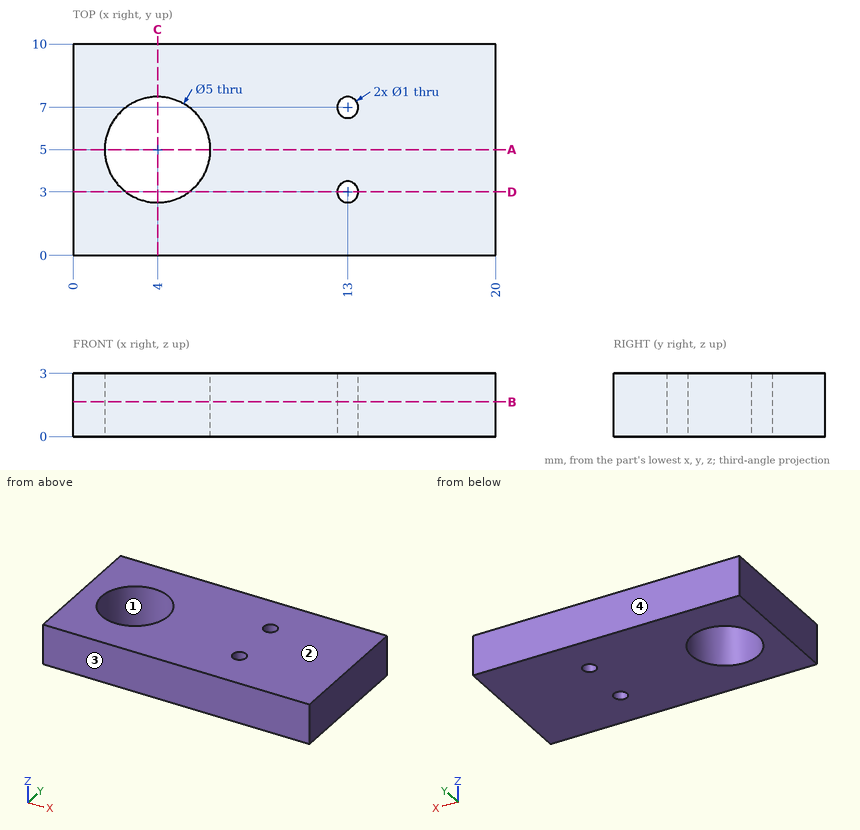
Can you work these out from the drawing? Everything is in mm from the part's minimum corner. Round coordinates to 2 decimals unless told otherwise and drop trailing zeros. Write each loop counter-clockwise with the first axis right and the second up, starting at its lowest first coordinate (ties: lowest second). Pieces come first, ordered by that corner, then holes. Notation, with made-up numbers: (62, 52.25) - (81, 52.25) arc R14 cw to (81, 59.25) - close; hole circle Ø8 at (46.5, -2.75). An arc over 180 degrees is marked (long way). Use a Markdown table: item, result.
Q1. I want a section at C-C (x = 4). List the corners of the cut face in (y, z) for me.
Output values:
| item | result |
|---|---|
| outline | (0, 0) - (2.5, 0) - (2.5, 3) - (0, 3) - close; (7.5, 0) - (10, 0) - (10, 3) - (7.5, 3) - close |
Q2. Please list where these lines run through material, in increasing order: L1, parallel to Y at x = 13, z = 2.2; L2, parallel to Y at x = 4, z = 1.4; L3, parallel to Y at x = 3.25, z = 0.65.
Output values:
| item | result |
|---|---|
| L1 | 0 to 2.5, 3.5 to 6.5, 7.5 to 10 |
| L2 | 0 to 2.5, 7.5 to 10 |
| L3 | 0 to 2.62, 7.38 to 10 |
Q3. I want a section at D-D (y = 3). List the corners of the cut face in (x, z) for me, plus the area to 3 significant figures.
Output values:
| item | result |
|---|---|
| outline | (0, 0) - (2.5, 0) - (2.5, 3) - (0, 3) - close; (5.5, 0) - (12.5, 0) - (12.5, 3) - (5.5, 3) - close; (13.5, 0) - (20, 0) - (20, 3) - (13.5, 3) - close |
| area | 48.0 mm2 |
Q4. I want a section at A-A (y = 5). List the corners of the cut face in (x, z) for me.
Output values:
| item | result |
|---|---|
| outline | (0, 0) - (1.5, 0) - (1.5, 3) - (0, 3) - close; (6.5, 0) - (20, 0) - (20, 3) - (6.5, 3) - close |
Q5. I want a section at B-B (z = 1.65). List the corners of the cut face in (x, y) for me.
Output values:
| item | result |
|---|---|
| outline | (0, 0) - (20, 0) - (20, 10) - (0, 10) - close; hole circle Ø5 at (4, 5); hole circle Ø1 at (13, 3); hole circle Ø1 at (13, 7) |
Q6. Thinking about a two-plate mould opening in Y: for the marked faces 1, 2, 3 and 4, which applies, released by +Y, released by -Y, zero draft, split by the parting line, or undercut?
Output values:
| item | result |
|---|---|
| face 1 | undercut |
| face 2 | zero draft |
| face 3 | released by -Y |
| face 4 | released by +Y |
